from build123d import *

# Parameters (mm, degrees)
SKETCH1_W                      = 100
SKETCH1_H                      = 100
BOSS_EXTRUDE1_DEPTH            = 1.66
FILLET1_R                      = 10
M4_CLEARANCE_HOLE1_D           = 4.5
M4_CLEARANCE_HOLE1_DEPTH       = 22.648063607
M4_CLEARANCE_HOLE1_CSINK_D     = 4.55
M4_CLEARANCE_HOLE1_CSINK_ANGLE = 90
M4_CLEARANCE_HOLE1_TIP         = 1.351936393


with BuildPart() as part:
    # Sketch1 → Boss-Extrude1 (new body)
    with BuildSketch(Plane(origin=(0, 0, 0), x_dir=(1, 0, 0), z_dir=(0, 1, 0))):
        Rectangle(SKETCH1_W, SKETCH1_H)
    extrude(amount=BOSS_EXTRUDE1_DEPTH)

    # Fillet1
    fillet1_edges = [part.edges().sort_by_distance(p)[0] for p in [
        (50, 0.83, 50),
        (-50, 0.83, 50),
        (-50, 0.83, -50),
        (50, 0.83, -50),
    ]]
    fillet(fillet1_edges, radius=FILLET1_R)

    # M4 Clearance Hole1
    with Locations(Plane(origin=(0, 1.66, 0), x_dir=(1, 0, 0), z_dir=(0, 1, 0))):
        with Locations((-40, 40), (-40, -40), (40, -40), (40, 40)):
            CounterSinkHole(M4_CLEARANCE_HOLE1_D / 2, M4_CLEARANCE_HOLE1_CSINK_D / 2, depth=M4_CLEARANCE_HOLE1_DEPTH, counter_sink_angle=M4_CLEARANCE_HOLE1_CSINK_ANGLE)
            with Locations((0, 0, -(M4_CLEARANCE_HOLE1_DEPTH + M4_CLEARANCE_HOLE1_TIP / 2))):  # 118° drill point
                Cone(0, M4_CLEARANCE_HOLE1_D / 2, M4_CLEARANCE_HOLE1_TIP, mode=Mode.SUBTRACT)


solid = part.part
Could you check a few things on this model? Use its own coordinates, in mm. Give positions to 0.01 mm unless a question says otherwise; leave off trailing zeros. One line per question, with ' | ' between items.
1. I'm going to push a flat-ended pin straight in: pin 1 (1.5 mm diameter, centred on x = 4.5, z = 30.5, fed in from -Y). Where does the tip first touch, or does it pass through?
Results:
pin 1: y = 0
2. If I drill on line 1 (X direction, y = 0.45, z = -40); line 2 (X direction, y = 1.1, z = -38.5), over which ranges is the centre line in solid material (lowest first)?
Results:
line 1: -50 to -42.25, -37.75 to 37.75, 42.25 to 50 | line 2: -50 to -41.68, -38.32 to 38.32, 41.68 to 50
3. We'd pull the mould along Z, two halves only. Please class faces 1 (the face through (-1, 1.66, -1)), 2 (the face through (-47.15, 0.84, 46.99)), 3 (the face through (40.29, 0.81, 37.77)): +Z half, -Z half, draft (parallel to the pull), parting line (faces both ways), or undercut.
Results:
face 1: draft | face 2: +Z half | face 3: undercut
